from build123d import *

# Parameters (mm, degrees)
SKETCH1_R           = 2.6
BOSS_EXTRUDE1_DEPTH = 4


with BuildPart() as part:
    # Sketch1 → Boss-Extrude1 (new body)
    with BuildSketch(Plane(origin=(0, 0, 0), x_dir=(1, 0, 0), z_dir=(0, 1, 0))):
        Polygon((0, 0), (60, 0), (60, 20), (20, 60), (0, 60), align=None)
        with Locations((10, 10)):
            Circle(SKETCH1_R, mode=Mode.SUBTRACT)
        with Locations((30, 10)):
            Circle(SKETCH1_R, mode=Mode.SUBTRACT)
        with Locations((50, 10)):
            Circle(SKETCH1_R, mode=Mode.SUBTRACT)
        with Locations((10, 30)):
            Circle(SKETCH1_R, mode=Mode.SUBTRACT)
        with Locations((10, 50)):
            Circle(SKETCH1_R, mode=Mode.SUBTRACT)
    extrude(amount=BOSS_EXTRUDE1_DEPTH)


solid = part.part
Could you check a few things on this model? Use its own coordinates, in mm. Give positions to 0.01 mm unless a question says otherwise; leave off trailing zeros. Order: outer loops, then holes, each group sorted by start corner. A loop starts at its lowest first (then second) coordinate and runs counter-clockwise, first axis right, second up. Notation, with made-up numbers: (-24.5, -26.5) - (27.5, -26.5) arc R24 cw to (27.5, -9.5) - close; hole circle Ø8 at (-6.75, 61.25). An arc over 180 degrees is marked (long way). One line per question, with ' | ' between items. Start each with the question number.
Item 1: I want a section at C-C on y = 1.9. Write out the boundary of the cut face in (x, z), then the cut area to 3 significant figures.
Item 2: I want a section at A-A on x = 10. Write out the boundary of the cut face in (y, z).
Item 3: I need wall thicknesses on probe 1 along Z at (x, y) = (10, 2.65); probe 2 along X at (y, z) = (1.75, -10); probe 3 along Z at (x, y) = (11.5, 2.55). Which ranges of each line are inside material? Lowest first, please. Write a range as [from, to].
Item 4: I want a section at D-D on x = 30. Write out the boundary of the cut face in (y, z), then the cut area to 3 significant figures.
Item 5: Thinking about a two-plate mould opening in Z: for faces 1 (the cylindrical face through (29.44, 1.97, -7.46)), 2 (the flat face through (0, 2, -30)), 3 (the flat face through (40, 2, -40)), which applies, pulls with the +Z half, pulls with the -Z half, needs draft (parallel to the pull), parting line crosses it, or undercut?
Item 6: I want a section at B-B on z = -10. Write out the boundary of the cut face in (x, y).
Verdict:
1) outline: (0, -60) - (20, -60) - (60, -20) - (60, 0) - (0, 0) - close; hole circle Ø5.2 at (10, -50); hole circle Ø5.2 at (10, -30); hole circle Ø5.2 at (10, -10); hole circle Ø5.2 at (30, -10); hole circle Ø5.2 at (50, -10) | area: 2,690 mm^2
2) outline: (0, -60) - (4, -60) - (4, -52.6) - (0, -52.6) - close; (0, -47.4) - (4, -47.4) - (4, -32.6) - (0, -32.6) - close; (0, -27.4) - (4, -27.4) - (4, -12.6) - (0, -12.6) - close; (0, -7.4) - (4, -7.4) - (4, 0) - (0, 0) - close
3) probe 1: [-60, -52.6], [-47.4, -32.6], [-27.4, -12.6], [-7.4, 0] | probe 2: [0, 7.4], [12.6, 27.4], [32.6, 47.4], [52.6, 60] | probe 3: [-60, -52.12], [-47.88, -32.12], [-27.88, -12.12], [-7.88, 0]
4) outline: (0, -50) - (4, -50) - (4, -12.6) - (0, -12.6) - close; (0, -7.4) - (4, -7.4) - (4, 0) - (0, 0) - close | area: 179 mm^2
5) face 1: undercut | face 2: needs draft | face 3: pulls with the -Z half
6) outline: (0, 0) - (7.4, 0) - (7.4, 4) - (0, 4) - close; (12.6, 0) - (27.4, 0) - (27.4, 4) - (12.6, 4) - close; (32.6, 0) - (47.4, 0) - (47.4, 4) - (32.6, 4) - close; (52.6, 0) - (60, 0) - (60, 4) - (52.6, 4) - close
